Read the model definition and answer for the solid it produces. Units are mm, in the model's axes. A direction names the side the tool comes from. Give positions to 0.01 mm unless a question says otherwise; leave off trailing zeros. Write each loop counter-clockwise with the first axis right and the second up, starting at its lowest first coordinate (ties: lowest second). Pieces come first, ordered by that corner, then holes. Notation, with made-up numbers: M -27,-24 L 11,-24 A19 cw 11,12 Z; hole C 51,86.5 d3. An arc over 180 degrees is marked long. Put each result on its own line as item: value.
from build123d import *

# Parameters (mm, degrees)
CROQUIS1_W              = 150
CROQUIS1_H              = 90
SALIENTE_EXTRUIR1_DEPTH = 24.5
CORTAR_EXTRUIR2_DEPTH   = 91.830886817
CROQUIS6_R              = 14.2875
CORTAR_EXTRUIR3_DEPTH   = 4.7625
CORTAR_EXTRUIR4_START   = -140
CROQUIS2_R              = 6.35
CROQUIS2_R_2            = 3.175
CORTAR_EXTRUIR4_DEPTH   = 5.2375
CORTAR_EXTRUIR1_DEPTH   = 41
SALIENTE_EXTRUIR2_START = 4.7625
SALIENTE_EXTRUIR2_DEPTH = 4.7625
CROQUIS8_W              = 60
CROQUIS8_H              = 10
SALIENTE_EXTRUIR3_DEPTH = 0.1


with BuildPart() as part:
    # Croquis1 → Saliente-Extruir1 (new body)
    with BuildSketch(Plane(origin=(0, 0, 0), x_dir=(1, 0, 0), z_dir=(0, 1, 0))):
        Rectangle(CROQUIS1_W, CROQUIS1_H)
    extrude(amount=SALIENTE_EXTRUIR1_DEPTH)

    # Croquis3 → Cortar-Extruir2 (cut, through all)
    with BuildSketch(Plane(origin=(0, 24.5, 0), x_dir=(1, 0, 0), z_dir=(0, 1, 0))):
        with BuildLine():
            Line((58.65, -25), (-58.65, -25))
            ThreePointArc((-58.65, -25), (-63.140128061, -23.140128061), (-65, -18.65))
            Line((-65, -18.65), (-65, 18.65))
            ThreePointArc((-65, 18.65), (-63.140128061, 23.140128061), (-58.65, 25))
            Line((-58.65, 25), (58.65, 25))
            ThreePointArc((58.65, 25), (63.140128061, 23.140128061), (65, 18.65))
            Line((65, 18.65), (65, -18.65))
            ThreePointArc((65, -18.65), (63.140128061, -23.140128061), (58.65, -25))
        make_face()
        with BuildLine():
            Line((-75, -45), (-30, -45))
            Line((-30, -45), (-30, -41.35))
            ThreePointArc((-30, -41.35), (-31.859871939, -36.859871939), (-36.35, -35))
            Line((-36.35, -35), (-75, -35))
            Line((-75, -35), (-75, -45))
        make_face()
        with BuildLine():
            Line((75, -45), (30, -45))
            Line((30, -45), (30, -41.35))
            ThreePointArc((30, -41.35), (31.859871939, -36.859871939), (36.35, -35))
            Line((36.35, -35), (75, -35))
            Line((75, -35), (75, -45))
        make_face()
        with BuildLine():
            Line((-45, 45), (45, 45))
            Line((45, 45), (45, 41.35))
            ThreePointArc((45, 41.35), (43.140128061, 36.859871939), (38.65, 35))
            Line((38.65, 35), (-38.65, 35))
            ThreePointArc((-38.65, 35), (-43.140128061, 36.859871939), (-45, 41.35))
            Line((-45, 41.35), (-45, 45))
        make_face()
    extrude(amount=-CORTAR_EXTRUIR2_DEPTH, mode=Mode.SUBTRACT)

    # Croquis6 → Cortar-Extruir3 (cut)
    with BuildSketch(Plane.ZY.offset(75)):
        with Locations((0.019345319, 12.255943197)):
            Circle(CROQUIS6_R)
    extrude(amount=-CORTAR_EXTRUIR3_DEPTH, mode=Mode.SUBTRACT)

    # Croquis2 → Cortar-Extruir4 (cut)
    with BuildSketch(Plane(origin=(75, 0, 0), x_dir=(0, 0, -1), z_dir=(1, 0, 0)).offset(CORTAR_EXTRUIR4_START)):
        with Locations(Location((-0.019345319, 12.255943197, 0), (0, 0, 180))):
            Circle(CROQUIS2_R)
        with Locations(Location((-20.019346202, 12.25, 0), (0, 0, 64.450536277))):
            Circle(CROQUIS2_R_2)
        with Locations(Location((19.980653798, 12.25, 0), (0, 0, 114.778004308))):
            Circle(CROQUIS2_R_2)
    extrude(amount=-CORTAR_EXTRUIR4_DEPTH, mode=Mode.SUBTRACT)

    # Croquis2 → Cortar-Extruir1 (cut)
    with BuildSketch(Plane(origin=(75, 0, 0), x_dir=(0, 0, -1), z_dir=(1, 0, 0))):
        with Locations(Location((-0.019345319, 12.255943197, 0), (0, 0, 180))):
            Circle(CROQUIS2_R)
        with Locations(Location((-20.019346202, 12.25, 0), (0, 0, 64.450536277))):
            Circle(CROQUIS2_R_2)
        with Locations(Location((19.980653798, 12.25, 0), (0, 0, 114.778004308))):
            Circle(CROQUIS2_R_2)
    extrude(amount=-CORTAR_EXTRUIR1_DEPTH, mode=Mode.SUBTRACT)

    # Croquis7 → Saliente-Extruir2 (add)
    with BuildSketch(Plane.ZY.offset(75).offset(SALIENTE_EXTRUIR2_START)):
        with BuildLine():
            Line((-12.18478223, 24.5), (-7.343787794, 24.5))
            ThreePointArc((-7.343787794, 24.5), (-14.268150014, 12.244395432), (-7.323985846, 0))
            Line((-7.323985846, 0), (-12.172845321, 0))
            ThreePointArc((-12.172845321, 0), (-17.268152629, 12.247520368), (-12.18478223, 24.5))
        make_face()
        with BuildLine():
            Line((7.382478433, 24.5), (12.223472869, 24.5))
            ThreePointArc((12.223472869, 24.5), (17.306843268, 12.247520368), (12.21153596, 0))
            Line((12.21153596, 0), (7.362676485, 0))
            ThreePointArc((7.362676485, 0), (14.306840653, 12.244395432), (7.382478433, 24.5))
        make_face()
    extrude(amount=-SALIENTE_EXTRUIR2_DEPTH)

    # Croquis8 → Saliente-Extruir3 (add)
    with BuildSketch(Plane(origin=(0, 24.5, 0), x_dir=(1, 0, 0), z_dir=(0, 1, 0))):
        with Locations((0, -40)):
            Rectangle(CROQUIS8_W, CROQUIS8_H)
    extrude(amount=SALIENTE_EXTRUIR3_DEPTH)


solid = part.part
(1) Which of the six approach directions +Z, -Z, +X, -X, +Y, -Y give full straight-line access (tool end or side, diameter ignored) to faces 1 (the face through (-77.415, 12.438, 17.306)), 2 (the face through (-67.58, 13.23, 23.04)), 3 (the face through (-65, 18, 4))?
Result:
face 1: +Z, -X
face 2: none
face 3: +Y, -Y
(2) For a pull along X with two mould halves and no side action, classify faces 4 (the face through (-70.238, 12, -20)), 5 (the face through (-79.762, 11, 15)), 6 (the face through (69.13, 13.23, 23.04)), 7 (the face through (65, 18, 4)) as +X half, -X half, draft (parallel to the pull), parting line (faces both ways), or undercut.
Result:
face 4: undercut
face 5: -X half
face 6: draft
face 7: undercut
(3) Section C-C on z = 0.5 is taken. Determine the outline of the cut face in (x, y).
Result:
outline: M -70.24,0 L -65,0 L -65,5.92 L -70.24,5.92 Z; M -70.24,18.59 L -65,18.59 L -65,24.5 L -70.24,24.5 Z; M 65,0 L 75,0 L 75,5.92 L 65,5.92 Z; M 65,18.59 L 75,18.59 L 75,24.5 L 65,24.5 Z
(4) Straight lines are drawn through the part: line 1 along Z through (x, y) = (68.75, 12.25); line 2 along X through (y, z) = (19.75, 1.5); line 3 along Z through (x, y) = (14.5, 15.5). For each, find the intervals that lie inside material, in ascending order. Write a range as from..to.
Result:
line 1: z = -45..-23.16, -16.81..-6.33, 6.37..16.84, 23.19..35
line 2: x = -70.24..-65, 65..75
line 3: z = -35..-25, 25..45
(5) Section A-A on z = -37.5 is taken. Determine the outline of the cut face in (x, y).
Result:
outline: M -75,0 L -43.7,0 L -43.7,24.5 L -75,24.5 Z; M 43.7,0 L 75,0 L 75,24.5 L 43.7,24.5 Z
(6) Given pin 1 Ø5 at (y, z) = (11, 38) entering from -X; pin 2 Ø14.5 at (y, z) = (12.26, 0.02) entering from -X; pin 3 Ø5 at (y, z) = (10.5, 22) entering from -X; pin 4 Ø8 at (x, z) = (-22.5, 18.5) entering from +Y, each flat-ended and moving along its own axis, determine where each tip first touches the part or whether it passes through.
Result:
pin 1: stops at x = -33.88
pin 2: stops at x = -70.24
pin 3: stops at x = -75
pin 4: passes through
(7) Section B-B on x = -42 is taken. Determine the outline of the cut face in (y, z).
Result:
outline: M 0,-35.96 L 24.5,-35.96 L 24.5,-25 L 0,-25 Z; M 0,25 L 24.5,25 L 24.5,35 L 0,35 Z
